Job drawing, mm, ordinate dimensions from the low corner. One solid piece. A direction names the side the tool comes from. Round coordinates to 2 decimals unless told otherwise and drop trailing zeros. Loops run counter-clockwise (first coordinate to the right, second up) from the corner with the lowest first, then second, coordinate; pieces in that order, holes last. Notation, with made-up numbers: M 41,7 L 47,7 A15 cw 47,34 Z; hole C 7,11.5 d3. An arc over 180 degrees is marked long. Write each question's results on one line, items separated by ' | '. Start each with the question number.
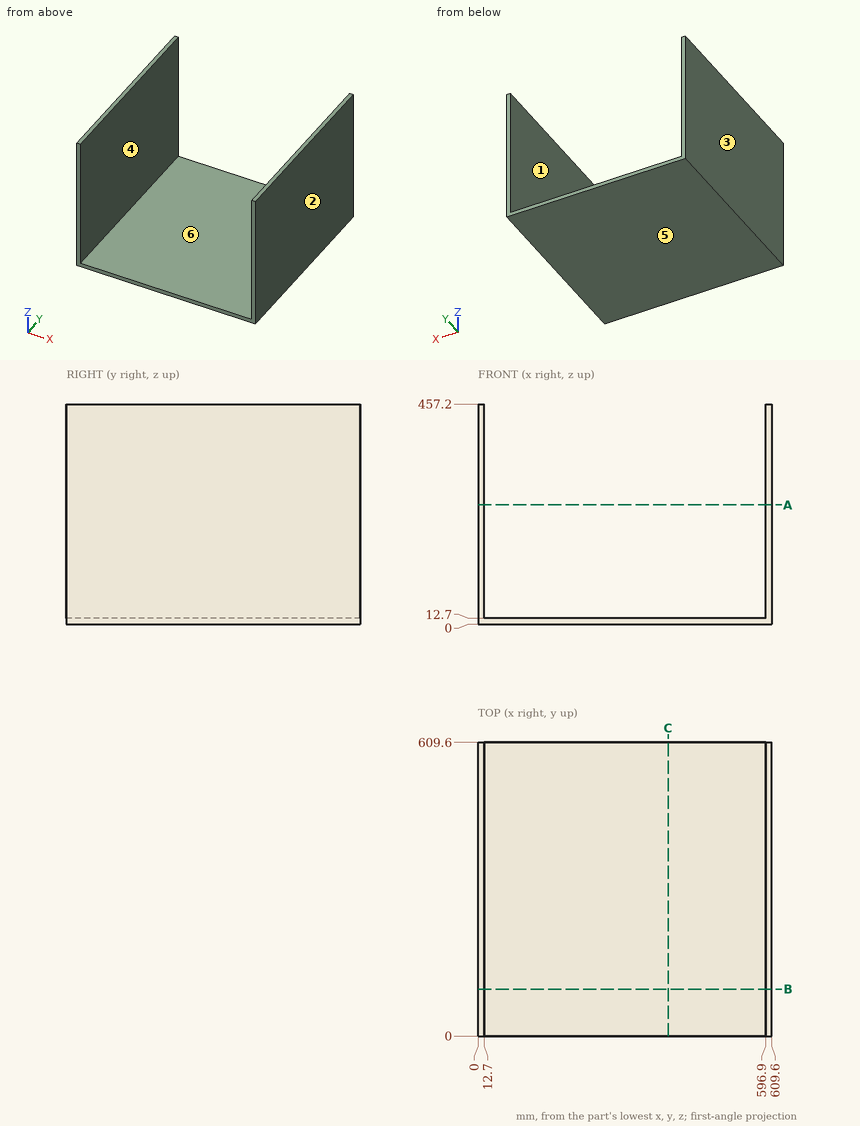
Item 1: Drop a flat-ended pin along its axis: pin 1 (10 mm diameter, centred on x = 432.5, y = 308, fed in from +Z). Give the stop position or say it passes through.
Item 2: Mould opens along X. For the marked faces 1, 2, 3 and 4 say: released by +X, released by -X, zero draft, split by the parting line, or undercut.
Item 3: Saw through at C-C, the plane x = 394.5. Give the cut face in (y, z), then the cut area to 3 significant figures.
Item 4: Saw through at A-A, the plane z = 248. Give the cut face in (x, y), then the cut area to 3 significant figures.
Item 5: Drill centre lines: line 1 along X through (y, z) = (31.5, 233.5); line 2 along Z through (x, y) = (51, 208). Where is each one in solid material? Low to high. Write a range as [from, to].
Item 6: Saw through at B-B, the plane y = 97.5. Give the cut face in (x, z).
Item 7: Tool access for the marked faces 5 and 6: list every direction of +Z, -Z, +X, -X, +Y, -Y with a clear straight run to the whole face (end or side of a thin tool).
Working result:
1) pin 1: stops at z = 12.7
2) face 1: undercut | face 2: released by +X | face 3: released by -X | face 4: undercut
3) outline: M 0,0 L 609.6,0 L 609.6,12.7 L 0,12.7 Z | area: 7,740 mm²
4) outline: M 0,0 L 12.7,0 L 12.7,609.6 L 0,609.6 Z; M 596.9,0 L 609.6,0 L 609.6,609.6 L 596.9,609.6 Z | area: 15,500 mm²
5) line 1: x = [0, 12.7], [596.9, 609.6] | line 2: z = [0, 12.7]
6) outline: M 0,0 L 609.6,0 L 609.6,457.2 L 596.9,457.2 L 596.9,12.7 L 12.7,12.7 L 12.7,457.2 L 0,457.2 Z
7) face 5: -Z, +X, -X, +Y, -Y | face 6: +Z, +Y, -Y
